The model under review builds one solid part; all positions refer to its coordinate system, in mm. Face numbers are marked on the shaded views. A direction names the side the tool comes from. Coordinates: 2 decimals unless noted, no trailing zeros. Loops run counter-clockwise (first coordinate to the right, second up) from the corner with the lowest first, then second, coordinate; pieces in that order, holes last. Notation, with made-up numbers: M 42.25,-29 L 79.25,-29 A24 ccw 79.25,10 Z; hole C 74,80.5 d3. An arc over 180 degrees is marked long. One line per item, written item: value.
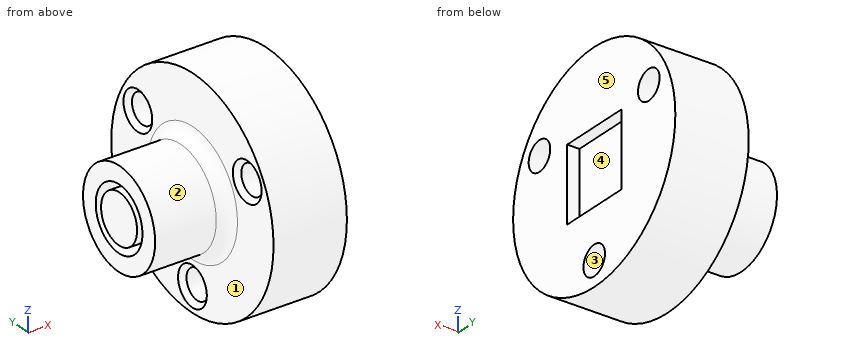
```python
from build123d import *

# Parameters (mm, degrees)
SKETCH3_W                       = 9.525
SKETCH3_H                       = 7.9375
SKETCH4_W                       = 9.525
SKETCH4_H                       = 9.525
CUT_EXTRUDE1_DEPTH              = 1.5875
FILLET1_R                       = 1.5875
F_6_CLEARANCE_HOLE1_D           = 3.7973
F_6_CLEARANCE_HOLE1_CSINK_D     = 5.0673
F_6_CLEARANCE_HOLE1_CSINK_ANGLE = 90


with BuildPart() as part:
    # Sketch3 → Revolve1 (revolve)
    with BuildSketch(Plane.XY, mode=Mode.PRIVATE) as revolve1_sk:
        Polygon((-19.05, 0), (0, 0), (0, 6.35), (-9.525, 6.35), (-19.05, 6.35), (-19.05, 4.1148), (-12.7, 4.1148), (-12.7, 3.175), (-19.05, 3.175), align=None)
        with Locations((-4.7625, 10.31875)):
            Rectangle(SKETCH3_W, SKETCH3_H)
    revolve(revolve1_sk.sketch.rotate(Axis((-35.206134047, 0, 0), (1, 0, 0)), 180), axis=Axis((-35.206134047, 0, 0), (1, 0, 0)))

    # Sketch4 → Cut-Extrude1 (cut)
    with BuildSketch(Plane(origin=(0, 0, 0), x_dir=(0, 0, -1), z_dir=(1, 0, 0))):
        Rectangle(SKETCH4_W, SKETCH4_H)
    extrude(amount=-CUT_EXTRUDE1_DEPTH, mode=Mode.SUBTRACT)

    # Fillet1
    fillet1_edges = [part.edges().sort_by_distance(p)[0] for p in [
        (-9.525, 6.35, 0),
    ]]
    fillet(fillet1_edges, radius=FILLET1_R)

    # 6 Clearance Hole1 (through all)
    with Locations(Plane.ZY.offset(9.525)):
        with Locations((-11.1125, 0), (5.577986509, 9.611124947), (5.556221618, -9.648822845)):
            CounterSinkHole(F_6_CLEARANCE_HOLE1_D / 2, F_6_CLEARANCE_HOLE1_CSINK_D / 2, counter_sink_angle=F_6_CLEARANCE_HOLE1_CSINK_ANGLE)


solid = part.part
```
(1) Draft analysis for pull direction Y (two halves, no side actions). For the marked faces 1, 2 and 3, state which applies: pulls with the +Y half, pulls with the -Y half, needs draft (parallel to the pull), parting line crosses it, or undercut.
Checks:
face 1: needs draft
face 2: parting line crosses it
face 3: undercut
(2) To check wall thickness, follow L1, parallel to Y at x = -14, z = 1; L2, parallel to X at y = -10, z = -4.5 (3 decimals); L3, parallel to Y at x = -13, z = 3.5. State the ranges of each line that lie inside material, in increasing order. Write a range as [from, to].
Checks:
L1: [-6.27, -3.99], [-3.01, 3.01], [3.99, 6.27]
L2: [-9.525, 0]
L3: [-5.3, -2.16], [2.16, 5.3]
(3) Add section C-C on x = -7.5. State the section outline as (y, z) points (1 decimal).
Checks:
outline: C 0,0 d28.6; hole C -9.6,5.6 d3.8; hole C 0,-11.1 d3.8; hole C 9.6,5.6 d3.8
(4) Insertion check: pin 1 Ø5 at (y, z) = (0, -11.11) entering from -X; pin 2 Ø4.5 at (y, z) = (-9.65, 5.56) entering from -X; pin 3 Ø6 at (x, z) = (-5.5, -10.5) entering from -Y; pin 4 Ø3.5 at (y, z) = (9.61, 5.58) entering from -X. Each pin has a flat end and moves straight along its axis. Give the tip position at first contact, or say it passes through.
Checks:
pin 1: x = -9.49
pin 2: x = -9.25
pin 3: y = -12.16
pin 4: through
(5) Tool access review of the marked faces 4 and 5: name each direction out of +Z, -Z, +X, -X, +Y, -Y from which nothing blocks a thin tool from reaching the whole face with its end or side.
Checks:
face 4: +X
face 5: +Z, -Z, +X, +Y, -Y
